```python
from build123d import *

# Parameters (mm, degrees)
EXTRUDE_1_DEPTH      = 10
EXTRUDE_1_DEPTH_BACK = 0.044975992
SKETCH_1_W           = 104
SKETCH_1_H           = 44
EXTRUDE_2_DEPTH      = 44
CUT_EXTRUDE_1_DEPTH  = 44
CHAMFER_4_SIZE       = 4
SKETCH_9_W           = 30
SKETCH_9_H           = 10
CUT_EXTRUDE_5_DEPTH  = 10.044975992
CUT_EXTRUDE_6_REACH  = 81.761
SKETCH_10_W          = 10
SKETCH_10_H          = 2
CUT_EXTRUDE_8_REACH  = 73.006
FILLET_1_R           = 2
CHAMFER_6_SIZE       = 1
CUT_EXTRUDE_9_DEPTH  = 44


with BuildPart() as part:
    # 草图1 → 凸台-拉伸1 (new, two sides: drawn at the far end of the back side and taken through both)
    with BuildSketch(Plane(origin=(0, 0, 0), x_dir=(1, 0, 0), z_dir=(0, 1, 0)).offset(-EXTRUDE_1_DEPTH_BACK)):
        Rectangle(SKETCH_1_W, SKETCH_1_H)
    extrude(amount=EXTRUDE_1_DEPTH + EXTRUDE_1_DEPTH_BACK)

    # 草图2 → 凸台-拉伸2 (add)
    with BuildSketch(Plane(origin=(0, 0, -22), x_dir=(-1, 0, 0), z_dir=(0, 0, -1))):
        Polygon((12, -20.044975992), (12, -10.044975992), (2, -10.044975992), (2, -0.044975992), (-8, -0.044975992), (-8, -10.525129165), (-8, -20.044975992), align=None)
    extrude(amount=-EXTRUDE_2_DEPTH)

    # 草图3 → 切除-拉伸1 (cut)
    with BuildSketch(Plane.XY.offset(22)):
        with BuildLine():
            Line((-44.05, 4.977512004), (-37.95, 4.977512004))
            ThreePointArc((-37.95, 4.977512004), (-37.950409974, 5.027518726), (-37.951639785, 5.077512004))
            Line((-37.951639785, 5.077512004), (-44.048360215, 5.077512004))
            ThreePointArc((-44.048360215, 5.077512004), (-44.049590026, 5.027518726), (-44.05, 4.977512004))
        make_face()
        with BuildLine():
            ThreePointArc((-37.951639785, 4.877512004), (-37.950409974, 4.927505282), (-37.95, 4.977512004))
            Line((-37.95, 4.977512004), (-44.05, 4.977512004))
            ThreePointArc((-44.05, 4.977512004), (-44.049590026, 4.927505282), (-44.048360215, 4.877512004))
            Line((-44.048360215, 4.877512004), (-37.951639785, 4.877512004))
        make_face()
        with BuildLine():
            ThreePointArc((-44.048360215, 4.877512004), (-41, 1.927512004), (-37.951639785, 4.877512004))
            Line((-37.951639785, 4.877512004), (-44.048360215, 4.877512004))
        make_face()
        with BuildLine():
            Line((-44.048360215, 5.077512004), (-37.951639785, 5.077512004))
            ThreePointArc((-37.951639785, 5.077512004), (-41, 8.027512004), (-44.048360215, 5.077512004))
        make_face()
        with BuildLine():
            Line((37.95, 4.977512004), (44.05, 4.977512004))
            ThreePointArc((44.05, 4.977512004), (44.049590026, 5.027518726), (44.048360215, 5.077512004))
            Line((44.048360215, 5.077512004), (37.951639785, 5.077512004))
            ThreePointArc((37.951639785, 5.077512004), (37.950409974, 5.027518726), (37.95, 4.977512004))
        make_face()
        with BuildLine():
            ThreePointArc((44.048360215, 4.877512004), (44.049590026, 4.927505282), (44.05, 4.977512004))
            Line((44.05, 4.977512004), (37.95, 4.977512004))
            ThreePointArc((37.95, 4.977512004), (37.950409974, 4.927505282), (37.951639785, 4.877512004))
            Line((37.951639785, 4.877512004), (44.048360215, 4.877512004))
        make_face()
        with BuildLine():
            ThreePointArc((37.951639785, 4.877512004), (41, 1.927512004), (44.048360215, 4.877512004))
            Line((44.048360215, 4.877512004), (37.951639785, 4.877512004))
        make_face()
        with BuildLine():
            Line((37.951639785, 5.077512004), (44.048360215, 5.077512004))
            ThreePointArc((44.048360215, 5.077512004), (41, 8.027512004), (37.951639785, 5.077512004))
        make_face()
    extrude(amount=-CUT_EXTRUDE_1_DEPTH, mode=Mode.SUBTRACT)

    # 倒角4
    chamfer_4_edges = [part.edges().sort_by_distance(p)[0] for p in [
        (-2, -0.044975992, 0),
        (8, -0.044975992, 0),
    ]]
    chamfer(chamfer_4_edges, length=CHAMFER_4_SIZE)

    # 草图9 → 切除-拉伸5 (cut)
    with BuildSketch(Plane.XZ.offset(0.044975992)):
        with Locations((37, 7.5)):
            Rectangle(SKETCH_9_W, SKETCH_9_H)
        with Locations((37, -7.5)):
            Rectangle(SKETCH_9_W, SKETCH_9_H)
    extrude(amount=-CUT_EXTRUDE_5_DEPTH, mode=Mode.SUBTRACT)

    # 切除-拉伸6: up to this face of the body (flat: up to its plane)
    cut_extrude_6_end = Plane(part.part.faces().sort_by_distance((-52, 4.977512004, 0))[0])
    # 草图10 → 切除-拉伸6 (cut, up to the picked face)
    with BuildSketch(Plane(origin=(22, 0, 0), x_dir=(0, 0, -1), z_dir=(1, 0, 0)), mode=Mode.PRIVATE) as cut_extrude_6_sk1:
        with Locations((-7.5, 9)):
            Rectangle(SKETCH_10_W, SKETCH_10_H)
    cut_extrude_6_tool1 = split(extrude(cut_extrude_6_sk1.sketch, amount=-CUT_EXTRUDE_6_REACH, mode=Mode.PRIVATE), bisect_by=cut_extrude_6_end, keep=Keep.BOTH, mode=Mode.PRIVATE)
    add(cut_extrude_6_tool1.solids().sort_by(Axis((22, 9, 7.5), (-1, 0, 0)))[0], mode=Mode.SUBTRACT)

    # 切除-拉伸8: up to this face of the body (flat: up to its plane)
    cut_extrude_8_end = Plane(part.part.faces().sort_by_distance((-0.039931558, 1.054666799, 22))[0])
    # 草图12 → 切除-拉伸8 (cut, up to the picked face)
    with BuildSketch(Plane(origin=(0, 0, -22), x_dir=(-1, 0, 0), z_dir=(0, 0, -1)), mode=Mode.PRIVATE) as cut_extrude_8_sk1:
        with BuildLine():
            Line((41, 10), (-43.55, 10))
            Line((-43.55, 10), (-43.55, 6.650832057))
            ThreePointArc((-43.55, 6.650832057), (-40.12678754, 7.899839843), (-37.95, 4.977512004))
            Line((-37.95, 4.977512004), (37.95, 4.977512004))
            ThreePointArc((37.95, 4.977512004), (38.843324317, 7.134187686), (41, 8.027512004))
            Line((41, 8.027512004), (41, 10))
        make_face()
    cut_extrude_8_tool1 = split(extrude(cut_extrude_8_sk1.sketch, amount=-CUT_EXTRUDE_8_REACH, mode=Mode.PRIVATE), bisect_by=cut_extrude_8_end, keep=Keep.BOTH, mode=Mode.PRIVATE)
    add(cut_extrude_8_tool1.solids().sort_by(Axis((0.637872, 7.552245, -22), (0, 0, 1)))[0], mode=Mode.SUBTRACT)

    # 圆角1
    fillet_1_edges = [part.edges().sort_by_distance(p)[0] for p in [
        (-52, 8, 7.5),
    ]]
    fillet(fillet_1_edges, radius=FILLET_1_R)

    # 倒角6
    chamfer_6_edges = [part.edges().sort_by_distance(p)[0] for p in [
        (47.775, 10, -22),
        (-46.5, 10, 22),
    ]]
    chamfer(chamfer_6_edges, length=CHAMFER_6_SIZE)

    # 草图13 → 切除-拉伸9 (cut)
    with BuildSketch(Plane.XY.offset(22)):
        with BuildLine():
            ThreePointArc((-37.95, 4.977512004), (-38.4675062, 3.277813455), (-39.844409938, 2.154904768))
            Line((-39.844409938, 2.154904768), (-32.95, 4.977512004))
            Line((-32.95, 4.977512004), (-37.95, 4.977512004))
        make_face()
    extrude(amount=-CUT_EXTRUDE_9_DEPTH, mode=Mode.SUBTRACT)


solid = part.part
```
Verification items for the finished model (mm, model axes). A direction names the side the tool comes from. Coordinates: 2 decimals unless noted, no trailing zeros. Loops run counter-clockwise (first coordinate to the right, second up) from the corner with the lowest first, then second, coordinate; pieces in that order, holes last. Notation, with made-up numbers: (46, -1) - (69, -1) arc R20 ccw to (69, 9) - close; hole circle Ø2 at (-27.75, 21.5). An arc over 180 degrees is marked (long way). Answer as a JSON object with one key per item and string values.
(1) Mould release check, pull along Z, two halves, no side actions. Record for faces 6 (the flat face through (0, -3, -22)), 7 (the flat face through (37, 4, -12.5)), 8 (the flat face through (43.55, 8, 17)): pulls with the +Z half, pulls with the -Z half, needs draft (parallel to the pull), parting line crosses it, or undercut.
Response:
{"face 6": "pulls with the -Z half", "face 7": "undercut", "face 8": "needs draft"}
(2) Cross-section at A-A, the plane x = 41. Record the boundary of the cut face in (y, z).
Response:
{"outline": "(-0.04, -22) - (1.93, -22) - (1.93, -12.5) - (-0.04, -12.5) - close; (-0.04, -2.5) - (1.93, -2.5) - (1.93, 2.5) - (-0.04, 2.5) - close; (-0.04, 12.5) - (1.93, 12.5) - (1.93, 22) - (-0.04, 22) - close"}
(3) Go/stop test with flat-tipped pins: pin 1 Ø2 at (y, z) = (-2.5, 7.5) entering from +X (3 decimals); pin 2 Ø3 at (x, z) = (39, 2.5) entering from -Y (3 decimals); pin 3 Ø3 at (x, z) = (-4.5, -3) entering from +Y. Record where each tip stops, or that it passes through.
Response:
{"pin 1": "stops at x = 10.545", "pin 2": "stops at y = -0.045", "pin 3": "stops at y = 4.98"}
(4) Cross-section at B-B, the plane z = -11. Record the boundary of the cut face in (x, y).
Response:
{"outline": "(-52, -0.04) - (-6, -0.04) - (-2, -4.04) - (-2, -10.04) - (-12, -10.04) - (-12, -20.04) - (8, -20.04) - (8, -4.04) - (12, -0.04) - (22, -0.04) - (22, 4.98) - (-32.95, 4.98) - (-39.84, 2.15) arc R3.05 cw to (-44.05, 4.88) arc R3.05 cw to (-44.05, 5.08) arc R3.05 cw to (-41, 8.03) - (-41, 10) - (-52, 10) - close"}
(5) Access from +Z, -Z, +X, -X, +Y, -Y to the whole of each face (thin tool, end or side, straight path). Record for faces 1 (the flat face through (43.55, 8, 0)), 2 (the cylindrical face through (-51.43, 7.4, 7.43)), 3 (the flat face through (-12, -15, 0)), 4 (the flat face through (37, 4, 12.5)), 5 (the flat face through (-2, -7, 0)).
Response:
{"face 1": "+Z, -Z, +Y", "face 2": "-X, +Y", "face 3": "+Z, -Z, -X, -Y", "face 4": "+X, +Y, -Y", "face 5": "+Z, -Z, -X"}
(6) Cross-section at C-C, the plane y = -7.5. Record the boundary of the cut face in (x, z).
Response:
{"outline": "(-2, -22) - (8, -22) - (8, 22) - (-2, 22) - close"}
(7) Scan lines: line 1 along Y through (x, z) = (6, 12); line 2 along Y through (x, z) = (-33, 12); line 3 along X through (y, z) = (-13.5, 2). Record each from-to range of solid material in increasing order.
Response:
{"line 1": "y = -20.04 to 4.98", "line 2": "y = -0.04 to 4.96", "line 3": "x = -12 to 8"}
(8) Cross-section at D-D, the plane z = 11.5. Record the boundary of the cut face in (x, y).
Response:
{"outline": "(-52, -0.04) - (-6, -0.04) - (-2, -4.04) - (-2, -10.04) - (-12, -10.04) - (-12, -20.04) - (8, -20.04) - (8, -4.04) - (12, -0.04) - (22, -0.04) - (22, 4.98) - (-32.95, 4.98) - (-39.84, 2.15) arc R3.05 cw to (-44.05, 4.88) arc R3.05 cw to (-44.05, 5.08) arc R3.05 cw to (-41.41, 8) - (-50, 8) arc R2 ccw to (-52, 6) - close"}
